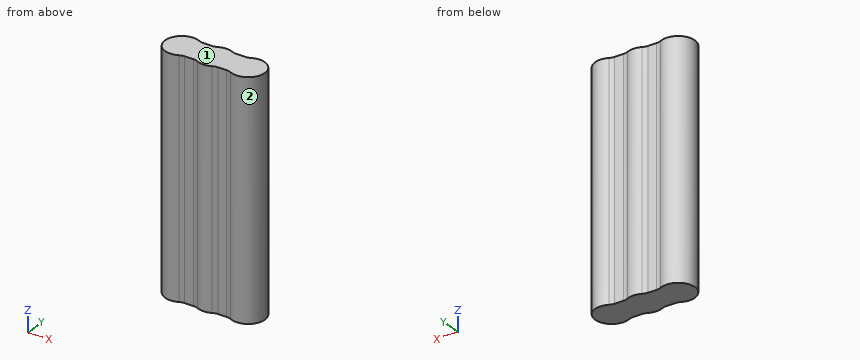
```python
from build123d import *

# Parameters (mm, degrees)
BOSS_EXTRUDE1_DEPTH = 129.3114


with BuildPart() as part:
    # Sketch1 → Boss-Extrude1 (new body)
    with BuildSketch(Plane.XY):
        with BuildLine():
            Line((3220.750449704, 2866.97511019), (3225.540701758, 2866.97511019))
            ThreePointArc((3225.540701758, 2866.97511019), (3226.972975907, 2867.138746899), (3228.331431905, 2867.621223336))
            ThreePointArc((3228.331431905, 2867.621223336), (3232.397525731, 2868.56261019), (3236.463619556, 2867.621223336))
            ThreePointArc((3236.463619556, 2867.621223336), (3237.822075555, 2867.138746899), (3239.254349704, 2866.97511019))
            Line((3239.254349704, 2866.97511019), (3244.044601758, 2866.97511019))
            ThreePointArc((3244.044601758, 2866.97511019), (3245.476875907, 2867.138746899), (3246.835331905, 2867.621223336))
            ThreePointArc((3246.835331905, 2867.621223336), (3260.153375731, 2859.31066019), (3246.835331905, 2851.000097044))
            ThreePointArc((3246.835331905, 2851.000097044), (3245.476875907, 2851.48257348), (3244.044601758, 2851.64621019))
            Line((3244.044601758, 2851.64621019), (3239.254349704, 2851.64621019))
            ThreePointArc((3239.254349704, 2851.64621019), (3237.822075555, 2851.48257348), (3236.463619556, 2851.000097044))
            ThreePointArc((3236.463619556, 2851.000097044), (3232.397525731, 2850.05871019), (3228.331431905, 2851.000097044))
            ThreePointArc((3228.331431905, 2851.000097044), (3226.972975907, 2851.48257348), (3225.540701758, 2851.64621019))
            Line((3225.540701758, 2851.64621019), (3220.750449704, 2851.64621019))
            ThreePointArc((3220.750449704, 2851.64621019), (3219.318175555, 2851.48257348), (3217.959719556, 2851.000097044))
            ThreePointArc((3217.959719556, 2851.000097044), (3204.641675731, 2859.31066019), (3217.959719556, 2867.621223336))
            ThreePointArc((3217.959719556, 2867.621223336), (3219.318175555, 2867.138746899), (3220.750449704, 2866.97511019))
        make_face()
    extrude(amount=BOSS_EXTRUDE1_DEPTH)


solid = part.part
```
CAD build for the part. Positions are in the model's coordinates, mm. Face numbers are marked on the shaded views. Give positions to 0.01 mm unless a question says otherwise; leave off trailing zeros. Order: outer loops, then holes, each group sorted by start corner. A loop starts at its lowest first (then second) coordinate and runs counter-clockwise, first axis right, second up.
(1) Saw through at B-B, the plane y = 2863.75. Give the cut face in (x, z).
(2) Flat gauge pins, fed straight in: pin 1 (6 mm diameter, centred on y = 2852, z = 32.5, fed in from +X); pin 2 (4 mm diameter, centred on x = 3240.5, z = 38.5, fed in from +Y); pin 3 (6 mm diameter, centred on y = 2866, z = 112, fed in from -X). Where does each tip first touch, or does it go through?
(3) Saw through at A-A, the plane z = 14.5. Give the cut face in (x, y), then the cut area to 3 significant figures.
(4) Saw through at C-C, the plane x = 3252.5. Give the cut face in (y, z), then the cut area to 3 significant figures.
(5) Mould opens along X. For the marked faces 1 and 2 say: released by +X, released by -X, zero draft, split by the parting line, or undercut.
(6) Drill centre lines: L1, parallel to X at y = 2867.75, z = 69.5; L2, parallel to Y at x = 3225, z = 34.5; L3, parallel to X at y = 2860, z = 86.5. Where is each one in solid material? Low to high.
Results found:
1. outline: (3205.78, 0) - (3259.02, 0) - (3259.02, 129.31) - (3205.78, 129.31) - close
2. pin 1: stops at x = 3259.09
2. pin 2: stops at y = 2867.02
2. pin 3: stops at x = 3205.41
3. outline: (3217.96, 2851) arc R6.35 cw to (3220.75, 2851.65) - (3225.54, 2851.65) arc R6.35 cw to (3228.33, 2851) arc R9.25 ccw to (3236.46, 2851) arc R6.35 cw to (3239.25, 2851.65) - (3244.04, 2851.65) arc R6.35 cw to (3246.84, 2851) arc R9.25 ccw (long way) to (3246.84, 2867.62) arc R6.35 cw to (3244.04, 2866.98) - (3239.25, 2866.98) arc R6.35 cw to (3236.46, 2867.62) arc R9.25 ccw to (3228.33, 2867.62) arc R6.35 cw to (3225.54, 2866.98) - (3220.75, 2866.98) arc R6.35 cw to (3217.96, 2867.62) arc R9.25 ccw (long way) to start
3. area: 883 mm2
4. outline: (2850.2, 0) - (2868.42, 0) - (2868.42, 129.31) - (2850.2, 129.31) - close
4. area: 2,360 mm2
5. face 1: zero draft
5. face 2: undercut
6. L1: x = 3210.1 to 3217.69, 3228.61 to 3236.19, 3247.11 to 3254.69
6. L2: y = 2851.65 to 2866.98
6. L3: x = 3204.67 to 3260.13
